Build history of the part. All positions in model axes, mm. Give positions to 0.01 mm unless a question says otherwise; leave off trailing zeros. Loops run counter-clockwise (first coordinate to the right, second up) from the corner with the lowest first, then second, coordinate; pieces in that order, holes last. Notation, with made-up numbers: M -18.5,49 L 30.5,49 A14 cw 30.5,56 Z; hole C 66,56 d3. An arc over 180 degrees is marked long. Answer as a JSON object with one key per item and string values. Group by question number.
1. Slice it at B-B (z = 6.25). List the corners of the cut face in (x, y), then the cut area to 3 significant figures.
2. Drop flat-ended pins along their axis: pin 1 Ø1 at (x, z) = (-6, 5.5) entering from +Y; pin 2 Ø4 at (x, z) = (11, 1.5) entering from +Y; pin 3 Ø1.5 at (x, y) = (12.5, -15.5) entering from -Z. Give the stop position or say it passes through.
3. Slice it at A-A (z = 3.25). List the corners of the cut face in (x, y), then the cut area to 3 significant figures.
4. Drill centre lines: line 1 along Y through (x, z) = (0, 4.5); line 2 along Y through (x, z) = (12, 2.5); line 3 along Y through (x, z) = (14.5, 5.25). Where is each one in solid material? Low to high. Write a range as [from, to].
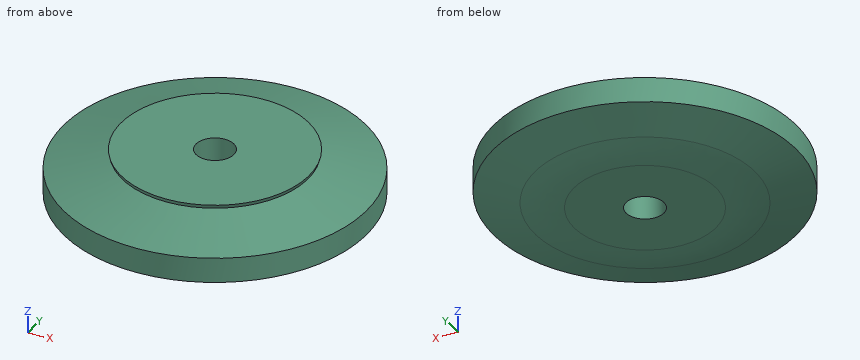
from build123d import *

# Parameters (mm, degrees)
F0_W = 5
F0_H = 1.6
F3_D = 5
F4_R = 20


with BuildPart() as f1:
    # F0 (on Front) → F1 (revolve)
    with BuildSketch(Plane.XZ):
        Polygon((0, 8), (0, 1.6), (5, 1.6), (10, 1.6), (10, 0), (12, 0), (20, 2.1435935394), (20, 5.446484726), (12.2725933897, 7.5170370869), (10.4701512597, 8), align=None)
        with Locations((2.5, 0.8)):
            Rectangle(F0_W, F0_H)
        Polygon((12.4020029122, 8), (10.4701512597, 8), (12.2725933897, 7.5170370869), align=None)
        with Locations((7.5, 0.8)):
            Rectangle(F0_W, F0_H)
    revolve(axis=Axis((0, 0, 4), (0, 0, 1)))

    # F3 (through all)
    with Locations(Plane.XY.offset(8)):
        with Locations((0, 0)):
            Hole(F3_D / 2)

    # F4
    f4_edges = [f1.edges().sort_by_distance(p)[0] for p in [
        (-12, 0, 0),
    ]]
    fillet(f4_edges, radius=F4_R)


solid = f1.part
Established:
{
 "1": {"outline": "C 0,0 d34; hole C 0,0 d5", "area": "888 mm^2"},
 "2": {"pin 1": "stops at y = 19.23", "pin 2": "stops at y = 17.81", "pin 3": "stops at z = 1.92"},
 "3": {"outline": "C 0,0 d40; hole C 0,0 d5", "area": "1,240 mm^2"},
 "4": {"line 1": "y = [-20, -2.5], [2.5, 20]", "line 2": "y = [-16, 16]", "line 3": "y = [-13.77, 13.77]"}
}
